Part model, mm, in its own coordinate system. Face numbers are marked on the shaded views. A direction names the side the tool comes from. Coordinates: 2 decimals unless noted, no trailing zeros. Loops run counter-clockwise (first coordinate to the right, second up) from the corner with the lowest first, then second, coordinate; pieces in that order, holes last. Notation, with made-up numbers: M 68,26 L 115,26 A12 cw 115,34 Z; hole C -15.5,36.5 d6. An arc over 180 degrees is marked long. Answer as a JSON object with one key per item and string values. Group by question number.
1. Drill centre line: L1, parallel to Y at x = 54.5, z = 5.5. Where is it in solid material? Low to high.
2. Saw through at C-C on z = 71.5. Count the separate pieces of the cut face and the enclosed holes in it, then the cut area to 3 significant figures.
3. Saw through at B-B on x = 38. Write the cut outline in (y, z).
4. Drop flat-ended pins along their axis: pin 1 Ø2 at (x, z) = (77, 27.5) entering from +Y; pin 2 Ø4.5 at (x, z) = (-77, 30.5) entering from -Y; pin 3 Ø4.5 at (x, z) = (-77, 27.5) entering from +Y. Give the stop position or say it passes through.
5. Saw through at A-A on y = 0. Write the cut outline in (x, z), then the cut area to 3 significant figures.
6. 3-axis set-ups, long thin cutter, end or side, ignore diameter. For the marked faces 5 and 6: which of +Z, -Z, +X, -X, +Y, -Y reach the whole face in a straight line?
7. Mould opens along Y. For the marked faces 1, 2, 3 and 4 say: released by +Y, released by -Y, zero draft, split by the parting line, or undercut.
from build123d import *

# Parameters (mm, degrees)
BOSS_EXTRU_1_DEPTH      = 110
ESQUISSE2_R             = 7.809149938
ENL_V_MAT_EXTRU_1_DEPTH = 159


with BuildPart() as part:
    # Esquisse1 → Boss.-Extru.1 (new body)
    with BuildSketch(Plane.XY):
        with BuildLine():
            Line((-79, 65), (-79, -65))
            ThreePointArc((-79, -65), (-74.899494937, -74.899494937), (-65, -79))
            Line((-65, -79), (65, -79))
            ThreePointArc((65, -79), (74.899494937, -74.899494937), (79, -65))
            Line((79, -65), (79, 65))
            ThreePointArc((79, 65), (74.899494937, 74.899494937), (65, 79))
            Line((65, 79), (-65, 79))
            ThreePointArc((-65, 79), (-74.899494937, 74.899494937), (-79, 65))
        make_face()
        with BuildLine():
            Line((-65, 75), (65, 75))
            ThreePointArc((65, 75), (72.071067812, 72.071067812), (75, 65))
            Line((75, 65), (75, -65))
            ThreePointArc((75, -65), (72.071067812, -72.071067812), (65, -75))
            Line((65, -75), (-65, -75))
            ThreePointArc((-65, -75), (-72.071067812, -72.071067812), (-75, -65))
            Line((-75, -65), (-75, 65))
            ThreePointArc((-75, 65), (-72.071067812, 72.071067812), (-65, 75))
        make_face(mode=Mode.SUBTRACT)
    extrude(amount=BOSS_EXTRU_1_DEPTH)

    # Esquisse2 → Enlèv. mat.-Extru.1 (cut, through all)
    with BuildSketch(Plane.ZY.offset(79)):
        with Locations((55, 0)):
            Circle(ESQUISSE2_R)
        with BuildLine():
            Line((22.964069625, 6.296228474), (35.649419661, 6.296228474))
            ThreePointArc((35.649419661, 6.296228474), (41.945648134, 0), (35.649419661, -6.296228474))
            Line((35.649419661, -6.296228474), (22.964069625, -6.296228474))
            ThreePointArc((22.964069625, -6.296228474), (16.667841152, 0), (22.964069625, 6.296228474))
        make_face()
        with BuildLine():
            Line((51.088422202, 32.413621937), (55.008410942, 20.349137125))
            ThreePointArc((55.008410942, 20.349137125), (50.965983423, 12.415426408), (43.032272706, 16.457853927))
            Line((43.032272706, 16.457853927), (39.112283966, 28.52233874))
            ThreePointArc((39.112283966, 28.52233874), (43.154711485, 36.456049456), (51.088422202, 32.413621937))
        make_face()
        with BuildLine():
            Line((84.618442346, 13.736491582), (74.355778588, 6.280229911))
            ThreePointArc((74.355778588, 6.280229911), (65.56119251, 7.673155505), (66.954118104, 16.467741582))
            Line((66.954118104, 16.467741582), (77.216781862, 23.924003253))
            ThreePointArc((77.216781862, 23.924003253), (86.011367939, 22.53107766), (84.618442346, 13.736491582))
        make_face()
        with BuildLine():
            Line((77.216781862, -23.924003253), (66.954118104, -16.467741582))
            ThreePointArc((66.954118104, -16.467741582), (65.56119251, -7.673155505), (74.355778588, -6.280229911))
            Line((74.355778588, -6.280229911), (84.618442346, -13.736491582))
            ThreePointArc((84.618442346, -13.736491582), (86.011367939, -22.53107766), (77.216781862, -23.924003253))
        make_face()
        with BuildLine():
            Line((39.112283966, -28.52233874), (43.032272706, -16.457853927))
            ThreePointArc((43.032272706, -16.457853927), (50.965983423, -12.415426408), (55.008410942, -20.349137125))
            Line((55.008410942, -20.349137125), (51.088422202, -32.413621937))
            ThreePointArc((51.088422202, -32.413621937), (43.154711485, -36.456049456), (39.112283966, -28.52233874))
        make_face()
    extrude(amount=-ENL_V_MAT_EXTRU_1_DEPTH, mode=Mode.SUBTRACT)


solid = part.part
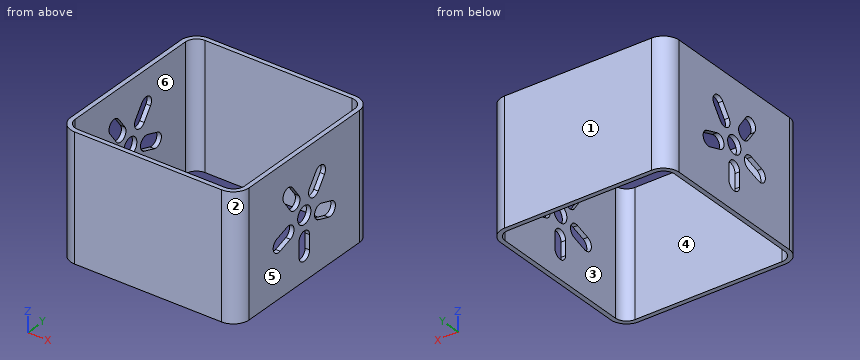
Outcome:
{
 "1": {"L1": "y = -79 to -75, 75 to 79"},
 "2": {"separate pieces": "4", "enclosed holes": "0", "area": "2,150 mm²"},
 "3": {"outline": "M -79,0 L -75,0 L -75,110 L -79,110 Z; M 75,0 L 79,0 L 79,110 L 75,110 Z"},
 "4": {"pin 1": "stops at y = 73.66", "pin 2": "stops at y = -75.05", "pin 3": "stops at y = 75.05"},
 "5": {"outline": "M -79,0 L -75,0 L -75,16.67 L -79,16.67 Z; M -79,41.95 L -75,41.95 L -75,47.19 L -79,47.19 Z; M -79,62.81 L -75,62.81 L -75,110 L -79,110 Z; M 75,0 L 79,0 L 79,16.67 L 75,16.67 Z; M 75,41.95 L 79,41.95 L 79,47.19 L 75,47.19 Z; M 75,62.81 L 79,62.81 L 79,110 L 75,110 Z", "area": "553 mm²"},
 "6": {"face 5": "+Z, -Z, +X, +Y, -Y", "face 6": "+Z, -Z"},
 "7": {"face 1": "released by +Y", "face 2": "released by -Y", "face 3": "undercut", "face 4": "undercut"}
}
